Read the model definition and answer for the solid it produces. Units are mm, in the model's axes. A direction names the side the tool comes from. Coordinates: 2 decimals unless noted, no trailing zeros. Loops run counter-clockwise (first coordinate to the right, second up) from the corner with the lowest first, then second, coordinate; pieces in that order, holes last. Notation, with made-up numbers: (16, 2.25) -> (62, 2.25) arc R16 ccw to (62, 15.25) -> close; hole circle Ø11 at (43.25, -28.75). An arc over 180 degrees is marked (long way). Answer as a JSON object with one key per item and string values. Group by question number.
1) Section A-A, the plane z = 0 is taken. Give the vertices of the cut face in (x, y).
2) Which of the six approach directions +Z, -Z, +X, -X, +Y, -Y give full straight-line access (tool end or side, diameter ignored) to faces 1 (the face through (-1.6, 0, 0)), 2 (the face through (1.521, -0.369, -7.327)), 3 (the face through (31.13, -1.28, -4.05))?
3) Section C-C, the plane y = 10.5 is taken. Give the vertices of the cut face in (x, z), plus the area to 3 significant figures.
4) Section D-D, the plane x = 11.5 is taken. Give the vertices of the cut face in (y, z), plus the area to 3 significant figures.
5) Consider probe 1 along Z at (x, y) = (1.75, 0); probe 2 along X at (y, z) = (-2, -8.75); probe 3 along Y at (x, z) = (2.2, 8.5). Determine where each line is inside the solid, lowest interval first. Write a range as [from, to].
6) Flat-ended cylindrical pins translate along their axes: P1, Ø10, axis at x = 18.5, z = 8, coming from the -Y side; P2, Ø3, axis at y = 0, z = -8.5, coming from the -X side; P3, Ø1.5, axis at x = 28, y = -7, coming from the -Z side. Find the tip coordinate at first contact, or state that the pin passes through.
7) Section B-B, the plane x = 2 is taken. Give the vertices of the cut face in (y, z).
8) Determine the mould class of faces 4 (the face through (32.3, 0, 0)), 5 (the face through (15.18, -12.19, -0.54)), 6 (the face through (1.521, -0.369, 9.673)) for opening direction Z: released by +Z, released by -Z, zero draft, split by the parting line, or undercut.
Autodesk Inventor part; units mm, degrees
ref_plane "YZ Plane" through (0, 0, 0) normal (1, 0, 0) x (0, 1, 0)
ref_plane "XZ Plane" through (0, 0, 0) normal (0, 1, 0) x (-1, 0, 0)
ref_plane "XY Plane" through (0, 0, 0) normal (0, 0, 1) x (1, 0, 0)
sketch "Szkic1" plane through (0, 0, 0) normal (1, 0, 0) x (0, 1, 0)
  circle A0 centre (0, 0) radius 12.2
  dimension "d0" = 24.4
extrude "Wyciągnięcie proste1" add sketch "Szkic1" along normal blind 30.8
sketch "Szkic2" plane through (30.8, 0, 0) normal (1, 0, 0) x (0, 0, -1)
  circle A0 centre (0, 0) radius 11.7
  dimension "d3" = 23.4
extrude "Wyciągnięcie proste2" cut sketch "Szkic2" against normal blind 0.8
sketch "Szkic3" plane through (30, 0, 0) normal (1, 0, 0) x (0, 0, -1)
  circle A0 centre (0, 0) radius 4.2479
extrude "Wyciągnięcie proste3" add sketch "Szkic3" along normal blind 2.3
sketch "Szkic4" plane through (0, 0, 0) normal (-1, 0, 0) x (0, 0, 1)
  line L0 (0, 0) -> (8.5, 0) construction
  line L1 (0, 0) -> (-8.5, 0) construction
  dimension "d8" = 8.5
hole "Otwór1" at (0, 0, 8.5) at (0, 0, -8.5) direction (1, 0, 0) diameter 2.459 depth 3 tip angle 118
sketch "Szkic5" plane through (0, 0, 0) normal (-1, 0, 0) x (0, 0, 1)
  circle A0 centre (0, 0) radius 3.2
  dimension "d16" = 6.4
extrude "Wyciągnięcie proste4" add sketch "Szkic5" along normal blind 1.6
properties part number "Silnik"
Determined:
{
 "1": {"outline": "(-1.6, -3.2) -> (0, -3.2) -> (0, -12.2) -> (30.8, -12.2) -> (30.8, -11.7) -> (30, -11.7) -> (30, -4.25) -> (32.3, -4.25) -> (32.3, 4.25) -> (30, 4.25) -> (30, 11.7) -> (30.8, 11.7) -> (30.8, 12.2) -> (0, 12.2) -> (0, 3.2) -> (-1.6, 3.2) -> close"},
 "2": {"face 1": "+Z, -Z, -X, +Y, -Y", "face 2": "-X", "face 3": "+X"},
 "3": {"outline": "(0, -6.21) -> (30.8, -6.21) -> (30.8, -5.16) -> (30, -5.16) -> (30, 5.16) -> (30.8, 5.16) -> (30.8, 6.21) -> (0, 6.21) -> close", "area": "374 mm²"},
 "4": {"outline": "circle Ø24.4 at (0, 0)", "area": "468 mm²"},
 "5": {"probe 1": "[-12.2, -9.73], [-7.27, 7.27], [9.73, 12.2]", "probe 2": "[0, 30]", "probe 3": "[-8.75, -1.23], [1.23, 8.75]"},
 "6": {"P1": "y = -11.83", "P2": "x = 0", "P3": "z = -10.48"},
 "7": {"outline": "circle Ø24.4 at (0, 0); hole circle Ø2.46 at (0, -8.5); hole circle Ø2.46 at (0, 8.5)"},
 "8": {"face 4": "zero draft", "face 5": "split by the parting line", "face 6": "undercut"}
}
